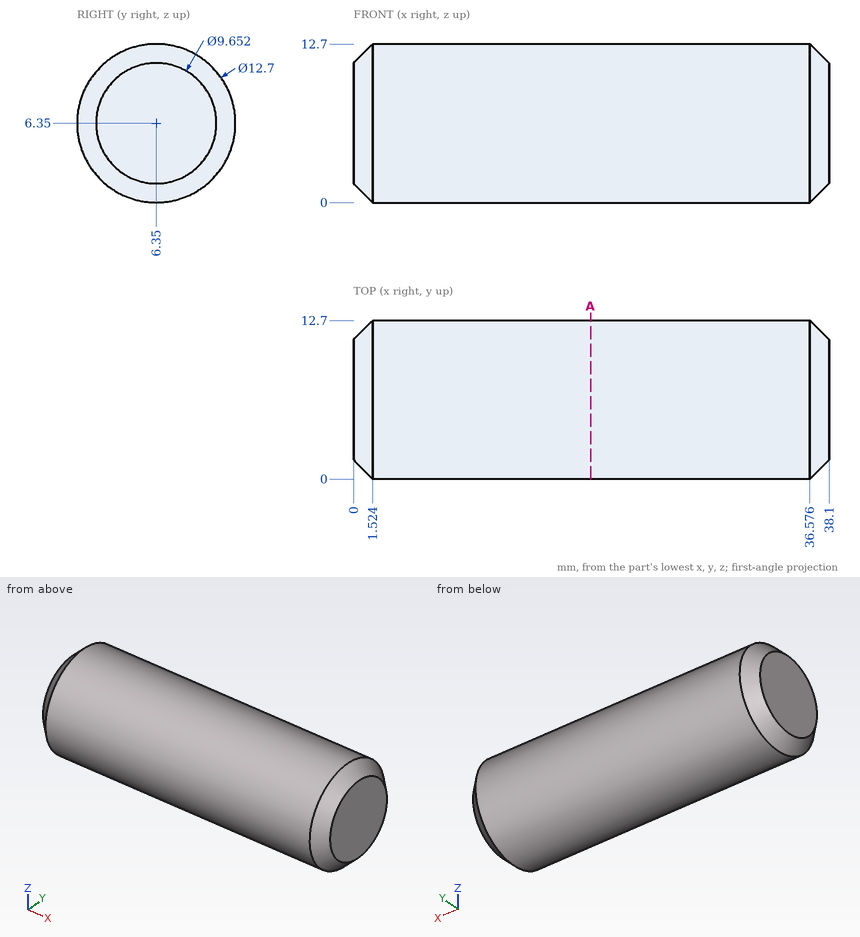
Geometry check sheet. Reference: drawing and pictorial views, mm from the part's lowest x, y, z. Give positions to 0.01 mm unless a question says otherwise; leave off trailing zeros. Order: outer loops, then holes, each group sorted by start corner. A loop starts at its lowest first (then second) coordinate and runs counter-clockwise, first axis right, second up. Notation, with made-up numbers: M 81,29 L 134,29 A31 ccw 134,57 Z; hole C 28,18 d9. An arc over 180 degrees is marked long. Answer in a Markdown table with one row per item. Add a question column.
Q1. Thickness scan on L1, parallel to Z at x = 21, y = 9.75; L2, parallel to Y at x = 9.5, z = 3.75; L3, parallel to X at y = 4.5, z = 0.5. Record the ranges inside material, lowest first.
Q2. Sectioned sample at A-A, the plane x = 19. Record the boundary of the cut face in (y, z), and give its area (3 significant figures).
Q3. Gauge pin test, flat ends, axial feed: pin 1 Ø1 at (x, z) = (23, 8.5) entering from +Y; pin 2 Ø2 at (x, y) = (7, 10) entering from -Z; pin 3 Ø4 at (x, y) = (27, 3.5) entering from +Z; pin 4 Ø4 at (x, z) = (4, 7.5) entering from -Y. Record the tip position at first contact, or that the pin passes through.
Verdict:
| question | item | result |
|---|---|---|
| 1 | L1 | 0.99 to 11.71 |
| 1 | L2 | 0.56 to 12.14 |
| 1 | L3 | 1.31 to 36.79 |
| 2 | outline | C 6.35,6.35 d12.7 |
| 2 | area | 127 mm² |
| 3 | pin 1 | y = 12.48 |
| 3 | pin 2 | z = 0.58 |
| 3 | pin 3 | z = 12.64 |
| 3 | pin 4 | y = 0 |
